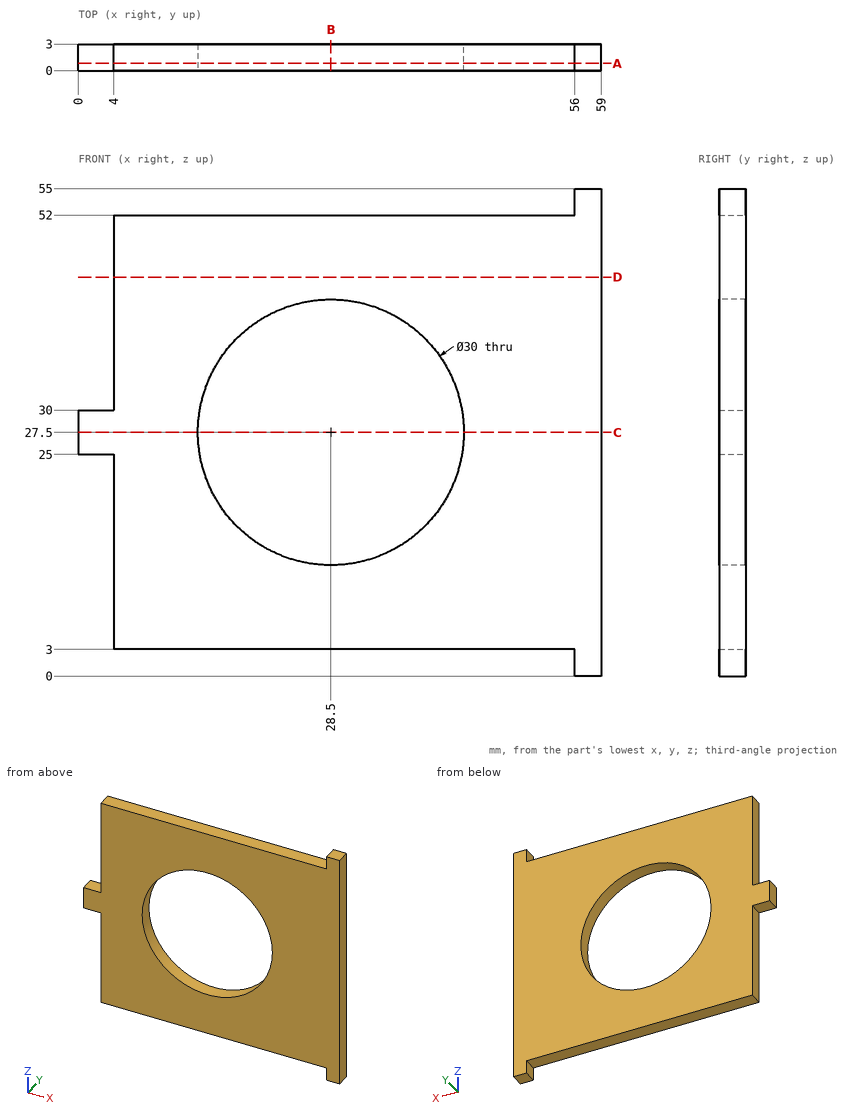
Source: three-view drawing plus pictorial views. Frame: mm from the lowest corner of the part. Round coordinates to 2 decimals unless told otherwise and drop trailing zeros. Loops run counter-clockwise (first coordinate to the right, second up) from the corner with the lowest first, then second, coordinate; pieces in that order, holes last.
Q1. Section C-C on z = 27.5. Return loops of the section in (x, y), plus the area to 3 significant figures.
Q2. Pin query (flat end, axial travel): P1, Ø1.5, axis at x = 43, z = 24, coming from the -Y side; P2, Ø0.9, axis at y = 2, z = 36, coming from the -X side; P3, Ø1.5, axis at y = 2, z = 54, coming from the -X side; P4, Ø0.9, axis at x = 3, y = 1, coming from the -Z side. Return the tip coordinate at first contact, or that it passes through.
Q3. Material intervals for L1, parallel to X at y = 1.45, z = 27.5; L2, parallel to Z at x = 28.5, y = 2.2; L3, parallel to Z at x = 46.5, y = 1.9, sorted ascending.
Q4. Section D-D on z = 45. Return loops of the section in (x, y), plus the area to 3 significant figures.
Q5. Section B-B on x = 28.5. Return loops of the section in (y, z).
Q6. Section A-A on y = 0.8. Return loops of the section in (x, z).
Evaluation:
1. outline: (0, 0) - (13.5, 0) - (13.5, 3) - (0, 3) - close; (43.5, 0) - (59, 0) - (59, 3) - (43.5, 3) - close
1. area: 87.0 mm2
2. P1: stops at y = 0
2. P2: stops at x = 4
2. P3: stops at x = 56
2. P4: stops at z = 25
3. L1: x = 0 to 13.5, 43.5 to 59
3. L2: z = 3 to 12.5, 42.5 to 52
3. L3: z = 3 to 52
4. outline: (4, 0) - (59, 0) - (59, 3) - (4, 3) - close
4. area: 165 mm2
5. outline: (0, 3) - (3, 3) - (3, 12.5) - (0, 12.5) - close; (0, 42.5) - (3, 42.5) - (3, 52) - (0, 52) - close
6. outline: (0, 25) - (4, 25) - (4, 3) - (56, 3) - (56, 0) - (59, 0) - (59, 55) - (56, 55) - (56, 52) - (4, 52) - (4, 30) - (0, 30) - close; hole circle Ø30 at (28.5, 27.5)
